Could you check a few things on this model? Use its own coordinates, in mm. A direction names the side the tool comes from. Give positions to 0.01 mm unless a question says otherwise; leave off trailing zeros. Loops run counter-clockwise (first coordinate to the right, second up) from the corner with the lowest first, then second, coordinate; pieces in that order, holes last. Notation, with made-up numbers: (-26.5, 78.5) - (-9.5, 78.5) arc R34 cw to (-9.5, 111.5) - close; hole circle Ø8 at (38, 15). An arc over 180 degrees is marked (long way). Answer in a Markdown table with one row per item. Add a question column.
```python
from build123d import *

# Parameters (mm, degrees)
SKETCH1_R           = 11
BOSS_EXTRUDE1_DEPTH = 10
SKETCH2_R           = 2.1
CUT_EXTRUDE1_DEPTH  = 58.089841478
CUT_EXTRUDE3_DEPTH  = 10
FILLET1_R           = 6
FILLET2_R           = 22


with BuildPart() as part:
    # Sketch1 → Boss-Extrude1 (new body)
    with BuildSketch(Plane(origin=(0, 0, 0), x_dir=(1, 0, 0), z_dir=(0, 1, 0))):
        with BuildLine():
            Line((-33, 0), (-45.5, 0))
            Line((-45.5, 0), (-43, -12))
            Line((-43, -12), (-32, -21))
            Line((-32, -21), (-13.747727085, -30))
            ThreePointArc((-13.747727085, -30), (27.772963416, 17.823089045), (-33, 0))
        make_face()
        with Locations(Location((-3.38, -0.39, 0), (0, 0, 270))):
            Circle(SKETCH1_R, mode=Mode.SUBTRACT)
    extrude(amount=BOSS_EXTRUDE1_DEPTH)

    # Sketch2 → Cut-Extrude1 (cut, through all)
    with BuildSketch(Plane(origin=(0, 10, 0), x_dir=(1, 0, 0), z_dir=(0, 1, 0))):
        with Locations(Location((9.62, 8.937379053, 0), (0, 0, 270))):
            Circle(SKETCH2_R)
        with Locations(Location((5.947379053, -13.39, 0), (0, 0, 270))):
            Circle(SKETCH2_R)
        with Locations(Location((-16.38, -9.717379053, 0), (0, 0, 270))):
            Circle(SKETCH2_R)
        with Locations(Location((-12.707379053, 12.61, 0), (0, 0, 270))):
            Circle(SKETCH2_R)
    extrude(amount=-CUT_EXTRUDE1_DEPTH, mode=Mode.SUBTRACT)

    # Sketch4 → Cut-Extrude3 (cut)
    with BuildSketch(Plane(origin=(0, 10, 0), x_dir=(1, 0, 0), z_dir=(0, 1, 0))):
        with BuildLine():
            ThreePointArc((-14.042553191, -23.644379879), (3.102926355, -27.324381933), (18.986679589, -19.893617021))
            ThreePointArc((18.986679589, -19.893617021), (19.118597761, -14.238301151), (13.46328189, -14.106382979))
            ThreePointArc((13.46328189, -14.106382979), (2.20025687, -19.375470825), (-9.957446809, -16.766014823))
            ThreePointArc((-9.957446809, -16.766014823), (-15.439182528, -18.16264416), (-14.042553191, -23.644379879))
        make_face()
        with BuildLine():
            ThreePointArc((18.186182669, 19.956521739), (6.35363251, 26.241786409), (-7.043478261, 26.065099539))
            ThreePointArc((-7.043478261, 26.065099539), (-9.861496228, 21.16012505), (-4.956521739, 18.342107083))
            ThreePointArc((-4.956521739, 18.342107083), (4.471074729, 18.466442288), (12.797684101, 14.043478261))
            ThreePointArc((12.797684101, 14.043478261), (18.448455124, 14.305750716), (18.186182669, 19.956521739))
        make_face()
    extrude(amount=-CUT_EXTRUDE3_DEPTH, mode=Mode.SUBTRACT)

    # Fillet1
    fillet1_edges = [part.edges().sort_by_distance(p)[0] for p in [
        (-33, 5, 0),
    ]]
    fillet(fillet1_edges, radius=FILLET1_R)

    # Fillet2
    # the kernel refuses this fillet: 22 mm, written as the material it takes off along each edge
    with BuildSketch(Plane(origin=(-13.747727085, -1.715684323, 30), x_dir=(0.913373582201966, 0, 0.4071224623323412), z_dir=(0, 1, 0))) as fillet2_piece_1:
        with BuildLine():
            CenterArc((0.45751582, 21.998810646), FILLET2_R, 267.776788076, 2.81898915)
            Line((-0.39592208, 0.015370429), (0, 0))
            ThreePointArc((0, 0), (0.343136865, -0.001784032), (0.686273729, 0))
        make_face()
    extrude(amount=13.431368647, mode=Mode.SUBTRACT)
    with BuildSketch(Plane(origin=(-32, -6.286877036, 21), x_dir=(-0.7739572992033206, 0, -0.6332377902572631), z_dir=(0, 1, 0))) as fillet2_piece_2:
        with BuildLine():
            CenterArc((FILLET2_R * 0.114306855208, -FILLET2_R), FILLET2_R, 90, 13.041994835)
            Line((-FILLET2_R * 0.111358301376, -FILLET2_R * 0.0257950743792), (0, 0))
            Line((0, 0), (FILLET2_R * 0.114306855208, 0))
        make_face()
    extrude(amount=22.573754073, mode=Mode.SUBTRACT)
    with BuildSketch(Plane(origin=(-43, -19.445362474, 12), x_dir=(-0.20395425411200122, 0, -0.978980419737605), z_dir=(0, 1, 0))) as fillet2_piece_3:
        with BuildLine():
            CenterArc((FILLET2_R * 0.353552044976, -FILLET2_R), FILLET2_R, 90, 38.942304205)
            Line((-FILLET2_R * 0.27498545547, -FILLET2_R * 0.222220718627), (0, 0))
            Line((0, 0), (FILLET2_R * 0.353552044976, 0))
        make_face()
    extrude(amount=48.890724947, mode=Mode.SUBTRACT)


solid = part.part
```
(1) We'd pull the mould along X, two halves only. Please class faces 1 (the cylindrical face through (4.341, 5.07, -18.497)), 2 (the cylindrical face through (29.44, 4.93, -14.91)), 3 (the cylindrical face through (18.388, 5.07, -14.241)), 4 (the flat face through (11, 10, 0)): pulls with the +X half, pulls with the -X half, needs draft (parallel to the pull), parting line crosses it, or undercut.
(2) Please list where these lines run through material, in increasing order: line 1 (Z direction, x = -15.5, y = 8.5); line 2 (X direction, y = 7.25, z = 13.39); line 3 (X direction, y = 4.75, z = 14).
(3) I want a section at D-D on z = 21. Please give me the cut outline in (x, y), then the cut area to 3 significant figures.
(4) I want a section at C-C on y = 4.75. Please give me the cut outline in (x, z), then the cut area to 3 significant figures.
(5) On a 3-axis mill with a long thin cutter (end or side, diameter ignored), from which of +Z, -Z, +X, -X, +Y, -Y can I reach the whole of each face in a straight line? I mean faces 5 (the flat face through (11, 0, 0)), 6 (the cylindrical face through (6.538, 5.07, -26.197)). Say none if no direction works.
(6) I want a section at B-B on x = -6. Please give me the cut outline in (y, z), then the cut area to 3 significant figures.
(7) For pin 1 Ø6 at (x, y) = (-24, 3.5) entering from -Z; pin 2 Ø5.5 at (x, y) = (-43, 6) entering from -Z; pin 3 Ø3 at (x, y) = (-13.5, 2) entering from +Z, each with a flat end and sliding along its axis, tell me the tip position at first contact or that it passes through.
(8) I want a section at A-A on z = -4. Please give me the cut outline in (x, y).
Reported:
| question | item | result |
|---|---|---|
| 1 | face 1 | undercut |
| 1 | face 2 | parting line crosses it |
| 1 | face 3 | undercut |
| 1 | face 4 | needs draft |
| 2 | line 1 | -29.13 to 7.81, 11.62 to 18.27, 22.14 to 29.14 |
| 2 | line 2 | -40.43 to 3.85, 8.05 to 14.5, 17.95 to 30.16 |
| 2 | line 3 | -39.94 to 3.94, 7.96 to 13.58, 18.87 to 29.88 |
| 3 | outline | (-31.73, 0) - (-15.92, 0) - (-15.92, 10) - (-31.73, 10) - close; (17.76, 0) - (25.46, 0) - (25.46, 10) - (17.76, 10) - close |
| 3 | area | 235 mm² |
| 4 | outline | (-45.5, 0) - (-38.54, 0) arc R6 cw to (-32.61, -5.08) arc R33 ccw (long way) to (-13.12, 30.28) arc R22 ccw to (-14.1, 29.82) - (-29.74, 22.11) arc R22 ccw to (-33.95, 19.41) - (-36.98, 16.93) arc R22 ccw to (-44.59, 4.39) - close; hole circle Ø4.2 at (-16.38, 9.72); hole circle Ø4.2 at (-12.71, -12.61); hole circle Ø22 at (-3.38, 0.39); hole (-14.04, 23.64) arc R4 ccw to (-9.96, 16.77) arc R19.5 cw to (13.46, 14.11) arc R4 ccw to (18.99, 19.89) arc R27.5 ccw to start; hole (-7.04, -26.07) arc R27 ccw to (18.19, -19.96) arc R4 ccw to (12.8, -14.04) arc R19 cw to (-4.96, -18.34) arc R4 ccw to start; hole circle Ø4.2 at (5.95, 13.39); hole circle Ø4.2 at (9.62, -8.94) |
| 4 | area | 2,700 mm² |
| 5 | face 5 | +Z, -Z, +X, -X, -Y |
| 5 | face 6 | +Y, -Y |
| 6 | outline | (0, -32.45) - (10, -32.45) - (10, -26.32) - (0, -26.32) - close; (0, -18.2) - (10, -18.2) - (10, -10.29) - (0, -10.29) - close; (0, 11.07) - (10, 11.07) - (10, 18.55) - (0, 18.55) - close; (0, 26.84) - (10, 26.84) - (10, 32.45) - (0, 32.45) - close |
| 6 | area | 271 mm² |
| 7 | pin 1 | z = -25.46 |
| 7 | pin 2 | z = 0 |
| 7 | pin 3 | z = 30.74 |
| 8 | outline | (-32.88, 0) - (-13.47, 0) - (-13.47, 10) - (-32.88, 10) - close; (6.71, 0) - (32.76, 0) - (32.76, 10) - (6.71, 10) - close |
